from build123d import *

# Parameters (mm, degrees)
PAD_DEPTH       = 20
SKETCH001_R     = 1.75
POCKET_DEPTH    = 32.88897
SKETCH002_R     = 5
POCKET001_DEPTH = 24
CHAMFER_SIZE    = 1.5
FILLET_R        = 1.5


with BuildPart() as part:
    # Sketch → Pad (new body)
    with BuildSketch(Plane.XY):
        with BuildLine():
            Line((-22.137351, -15.487065), (22.137351, -15.487065))
            Line((22.137351, 17.400905), (22.137351, -15.487065))
            Line((17.637351, 17.400905), (22.137351, 17.400905))
            ThreePointArc((-17.637351, 17.400905), (0, -5.538054), (17.637351, 17.400905))
            Line((-22.137351, 17.400905), (-17.637351, 17.400905))
            Line((-22.137351, -15.487065), (-22.137351, 17.400905))
        make_face()
    extrude(amount=PAD_DEPTH)

    # Sketch001 (on Face1 of Pad) → Pocket (cut, through all)
    with BuildSketch(Plane.XZ.offset(15.487065)):
        with Locations((-9.137351, 10)):
            Circle(SKETCH001_R)
        with Locations((9.137351, 10)):
            Circle(SKETCH001_R)
    extrude(amount=-POCKET_DEPTH, mode=Mode.SUBTRACT)

    # Sketch002 (on Face9 of Pocket) → Pocket001 (cut)
    with BuildSketch(Plane(origin=(0, 17.400905, 0), x_dir=(-1, 0, 0), z_dir=(0, 1, 0))):
        with Locations((-9.137351, 10)):
            Circle(SKETCH002_R)
        with Locations((9.137351, 10)):
            Circle(SKETCH002_R)
    extrude(amount=-POCKET001_DEPTH, mode=Mode.SUBTRACT)

    # Chamfer
    chamfer_edges = [part.edges().sort_by_distance(p)[0] for p in [
        (7.387351, -6.599095, 10),
        (-10.887351, -6.599095, 10),
    ]]
    chamfer(chamfer_edges, length=CHAMFER_SIZE)

    # Fillet
    fillet_edges = [part.edges().sort_by_distance(p)[0] for p in [
        (22.137351, 0.95692, 20),
        (19.887351, 17.400905, 20),
        (22.137351, 17.400905, 10),
        (19.887351, 17.400905, 0),
        (22.137351, 0.95692, 0),
        (-19.887351, 17.400905, 20),
        (-22.137351, 17.400905, 10),
        (-22.137351, 0.95692, 20),
        (-19.887351, 17.400905, 0),
        (-22.137351, 0.95692, 0),
    ]]
    fillet(fillet_edges, radius=FILLET_R)


solid = part.part
Input: part model. Units: mm. Frame: model coordinates. A direction names the side the tool comes from. Coordinates: 2 decimals unless noted, no trailing zeros. Loops run counter-clockwise (first coordinate to the right, second up) from the corner with the lowest first, then second, coordinate; pieces in that order, holes last. Notation, with made-up numbers: (66.5, 13) -> (89.5, 13) arc R18 ccw to (89.5, 29) -> close; hole circle Ø11 at (16.25, 2). An arc over 180 degrees is marked (long way). Write item = value, one per line. Start each with the question number.
Item 1: Reachability of faces 1 (the face through (5.87, -6.599, 8.96)), 2 (the face through (19, 17.401, 10)) from +Z, -Z, +X, -X, +Y, -Y: full face, straight path, thin tool, end or side. Return the list, or none.
Item 2: First-contact query: P1, Ø5, axis at x = -11, z = 8.5, coming from the +Y side; P2, Ø11.5, axis at x = -9.14, z = 10, coming from the +Y side; P3, Ø6, axis at x = 9.14, z = 10, coming from the +Y side. Flat tips, straight axial feed; report the tip coordinate or a pass-through.
Item 3: Cut plane B-B, the plane y = -11. Return loops of the section in (x, z).
Item 4: Cut plane C-C, the plane z = 2. Return loops of the section in (x, y).
Item 5: Cut plane D-D, the plane z = 10. Return loops of the section in (x, y).
Item 6: Material intervals for line 1 (X direction, y = -4.25, z = 10); line 2 (Y direction, x = 0, z = 9.75); line 3 (X direction, y = 4.5, z = 16.25), sorted ascending.
Item 7: Cut plane A-A, the plane y = 2. Return loops of the section in (x, z).
Item 8: Mould query, pull axis X, two halves, no side actions, for faces 3 (the face through (14.133, -3.523, 10.22)), 4 (the face through (-19.12, 16.95, 19.57)), 5 (the face through (21.69, -0.01, 0.43)). Classes: pulls with the +X half, pulls with the -X half, needs draft (parallel to the pull), parting line crosses it, or undercut.
Ans:
q1.face_1 = +Y
q1.face_2 = +Z, -Z, +X, -X, +Y
q2.P1 = -6.6
q2.P2 = 2.16
q2.P3 = -6.85
q3.outline = (-22.14, 1.5) arc R1.5 ccw to (-20.64, 0) -> (20.64, 0) arc R1.5 ccw to (22.14, 1.5) -> (22.14, 18.5) arc R1.5 ccw to (20.64, 20) -> (-20.64, 20) arc R1.5 ccw to (-22.14, 18.5) -> close; hole circle Ø3.5 at (-9.14, 10); hole circle Ø3.5 at (9.14, 10)
q4.outline = (-22.14, -15.49) -> (22.14, -15.49) -> (22.14, 15.9) arc R1.5 ccw to (20.64, 17.4) -> (17.64, 17.4) arc R18.25 cw (long way) to (-17.64, 17.4) -> (-20.64, 17.4) arc R1.5 ccw to (-22.14, 15.9) -> close
q5.outline = (-22.14, -15.49) -> (-10.89, -15.49) -> (-10.89, -8.1) -> (-12.39, -6.6) -> (-14.14, -6.6) -> (-14.14, 1.17) arc R18.25 cw to (-17.64, 17.4) -> (-20.64, 17.4) arc R1.5 ccw to (-22.14, 15.9) -> close; (-7.39, -15.49) -> (7.39, -15.49) -> (7.39, -8.1) -> (5.89, -6.6) -> (4.14, -6.6) -> (4.14, -5.06) arc R18.25 cw to (-4.14, -5.06) -> (-4.14, -6.6) -> (-5.89, -6.6) -> (-7.39, -8.1) -> close; (10.89, -15.49) -> (22.14, -15.49) -> (22.14, 15.9) arc R1.5 ccw to (20.64, 17.4) -> (17.64, 17.4) arc R18.25 cw to (14.14, 1.17) -> (14.14, -6.6) -> (12.39, -6.6) -> (10.89, -8.1) -> close
q6.line_1 = -22.14 to -14.14, 14.14 to 22.14
q6.line_2 = -15.49 to -5.54
q6.line_3 = -22.14 to -16.3, 16.3 to 22.14
q7.outline = (-22.14, 1.5) arc R1.5 ccw to (-20.64, 0) -> (-14.78, 0) -> (-14.78, 20) -> (-20.64, 20) arc R1.5 ccw to (-22.14, 18.5) -> close; (14.78, 0) -> (20.64, 0) arc R1.5 ccw to (22.14, 1.5) -> (22.14, 18.5) arc R1.5 ccw to (20.64, 20) -> (14.78, 20) -> close
q8.face_3 = undercut
q8.face_4 = needs draft
q8.face_5 = pulls with the +X half
